Geometry check sheet. Reference: drawing and pictorial views, mm from the part's lowest x, y, z. A direction names the side the tool comes from. Give positions to 0.01 mm unless a question says otherwise; leave off trailing zeros. Write each loop counter-clockwise with the first axis right and the second up, starting at its lowest first coordinate (ties: lowest second). Pieces come first, ordered by that corner, then holes. Notation, with made-up numbers: (37, -6.5) -> (80, -6.5) arc R21 cw to (80, 23.5) -> close; hole circle Ø1 at (-38, -9). An arc over 180 degrees is marked (long way). Use a Markdown table: item, result. Add a question column.
1. Cross-section at D-D (x = 34.5). Enter the section's corners in (y, z) (3 decimals), then the cut area to 3 significant figures.
2. Scan lines: probe 1 along X at (y, z) = (9.25, 10); probe 2 along Y at (x, z) = (30.5, 40) (3 decimals); probe 3 along X at (y, z) = (2.75, 65.5). Record each from-to range of solid material in increasing order. Write a range as [from, to].
3. Cross-section at B-B (x = 26). Enter the section's corners in (y, z) (3 decimals), then the cut area to 3 significant figures.
4. Release check for a two-part mould opening along Y. For the marked faces 1, 2 and 3 record: released by +Y, released by -Y, zero draft, split by the parting line, or undercut.
5. Cross-section at C-C (y = 8.25). Enter the section's corners in (x, z).
6. Cross-section at A-A (z = 64.5). Enter the section's corners in (x, y) (3 decimals), then the cut area to 3 significant figures.
7. Set-up check for the marked faces 4 and 5: record each of +Z, -Z, +X, -X, +Y, -Y from which the full face is reachable in a straight line by a thin tool's end or side.
8. Gauge pin test, flat ends, axial feed: P1, Ø1.3, axis at y = 7.5, z = 51.5, coming from the +X side; P2, Ø1, axis at y = 9.5, z = 52, coming from the -X side; P3, Ø17, axis at x = 33, z = 61.5, coming from the -Y side. Record the tip position at first contact, or that the pin passes through.
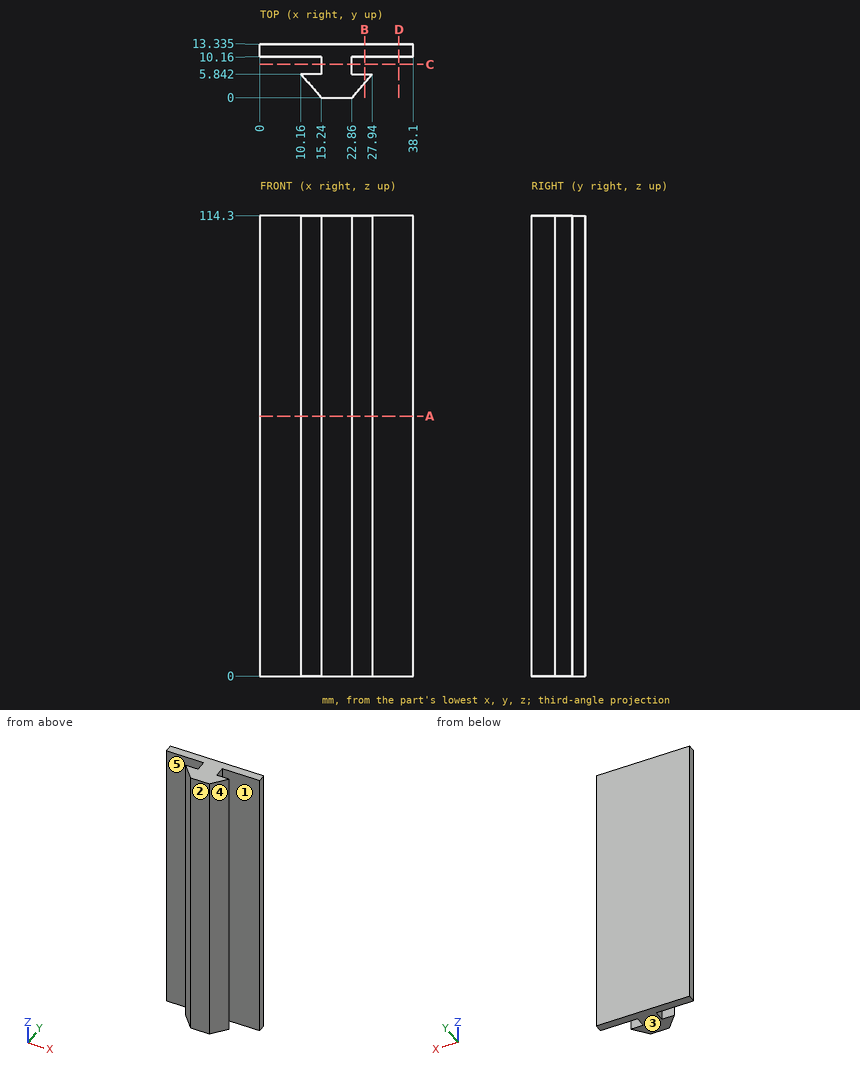
Worked answers:
| question | item | result |
|---|---|---|
| 1 | outline | (10.16, 0) -> (13.335, 0) -> (13.335, 114.3) -> (10.16, 114.3) -> close |
| 1 | area | 363 mm² |
| 2 | probe 1 | x = [15.24, 22.86] |
| 2 | probe 2 | y = [10.16, 13.335] |
| 2 | probe 3 | x = [12.85, 25.25] |
| 3 | outline | (3.611, 0) -> (5.842, 0) -> (5.842, 114.3) -> (3.611, 114.3) -> close; (10.16, 0) -> (13.335, 0) -> (13.335, 114.3) -> (10.16, 114.3) -> close |
| 3 | area | 618 mm² |
| 4 | face 1 | undercut |
| 4 | face 2 | released by -Y |
| 4 | face 3 | zero draft |
| 5 | outline | (15.24, 0) -> (22.86, 0) -> (22.86, 114.3) -> (15.24, 114.3) -> close |
| 6 | outline | (0, 10.16) -> (15.24, 10.16) -> (15.24, 5.842) -> (10.16, 5.842) -> (15.24, 0) -> (22.86, 0) -> (27.94, 5.842) -> (22.86, 5.842) -> (22.86, 10.16) -> (38.1, 10.16) -> (38.1, 13.335) -> (0, 13.335) -> close |
| 6 | area | 228 mm² |
| 7 | face 4 | +Z, -Z, +X, -Y |
| 7 | face 5 | +Z, -Z, -X |
| 8 | P1 | stops at x = 22.86 |
| 8 | P2 | stops at x = 15.24 |
| 8 | P3 | stops at y = 1.89 |
